The listing builds one solid part. Answer for the finished solid, in the listing's coordinates (mm). Face numbers are marked on the shaded views. A direction names the side the tool comes from. Coordinates: 2 decimals unless noted, no trailing zeros. Order: outer loops, then holes, each group sorted by start corner. A loop starts at its lowest first (then second) coordinate and runs counter-clockwise, first axis right, second up. Notation, with made-up numbers: (1.5, 4.5) -> (44.5, 4.5) arc R15 ccw to (44.5, 11.5) -> close; hole circle Ø8 at (-22.75, 55). An arc over 180 degrees is marked (long way). One line per question, with ' | ' between items.
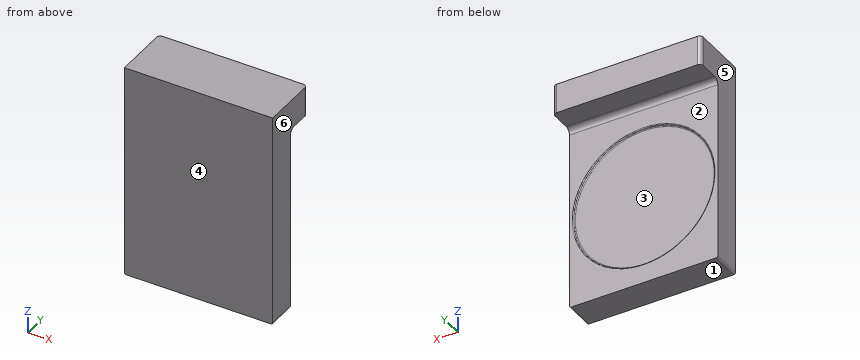
from build123d import *

# Parameters (mm, degrees)
SKETCH1_W           = 580
SKETCH1_H           = 80
BOSS_EXTRUDE1_DEPTH = 400
SKETCH2_W           = 400
SKETCH2_H           = 80
BOSS_EXTRUDE2_DEPTH = 75
FILLET2_R           = 10
FILLET3_R           = 5
FILLET4_R           = 15
SKETCH3_R           = 190
CUT_EXTRUDE1_DEPTH  = 5
FILLET6_R           = 2.5


with BuildPart() as part:
    # Sketch1 → Boss-Extrude1 (new body)
    with BuildSketch(Plane(origin=(0, 0, 0), x_dir=(0, 0, -1), z_dir=(1, 0, 0))):
        with Locations((290, 40)):
            Rectangle(SKETCH1_W, SKETCH1_H)
    extrude(amount=BOSS_EXTRUDE1_DEPTH)

    # Sketch2 → Boss-Extrude2 (add)
    with BuildSketch(Plane(origin=(0, 80, 0), x_dir=(1, 0, 0), z_dir=(0, 1, 0))):
        with Locations((200, 40)):
            Rectangle(SKETCH2_W, SKETCH2_H)
    extrude(amount=BOSS_EXTRUDE2_DEPTH)

    # Fillet2
    fillet2_edges = [part.edges().sort_by_distance(p)[0] for p in [
        (0, 155, -40),
        (400, 155, -40),
    ]]
    fillet(fillet2_edges, radius=FILLET2_R)

    # Fillet3
    fillet3_edges = [part.edges().sort_by_distance(p)[0] for p in [
        (400, 40, -580),
        (0, 40, -580),
    ]]
    fillet(fillet3_edges, radius=FILLET3_R)

    # Fillet4
    fillet4_edges = [part.edges().sort_by_distance(p)[0] for p in [
        (200, 80, -80),
    ]]
    fillet(fillet4_edges, radius=FILLET4_R)

    # Sketch3 → Cut-Extrude1 (cut)
    with BuildSketch(Plane(origin=(0, 80, 0), x_dir=(1, 0, 0), z_dir=(0, 1, 0))):
        with Locations(Location((200, 337.5, 0), (0, 0, 270))):
            Circle(SKETCH3_R)
    extrude(amount=-CUT_EXTRUDE1_DEPTH, mode=Mode.SUBTRACT)

    # Fillet6
    fillet6_edges = [part.edges().sort_by_distance(p)[0] for p in [
        (200, 75, -527.5),
        (200, 80, -527.5),
    ]]
    fillet(fillet6_edges, radius=FILLET6_R - 0.0001)  # a hair under: the kernel refuses the full size


solid = part.part
Item 1: Each of these flat-tipped pins is pushed along its axis until it touches: pin 1 Ø5 at (x, z) = (109, -120.5) entering from +Y; pin 2 Ø10 at (x, y) = (128, 94.5) entering from -Z. Where does it stop, or does it pass through?
Computed values:
pin 1: stops at y = 80 | pin 2: stops at z = -81.04
Item 2: Determine the mould class of the marked faces 3, 4, 5 and 6 for opening direction X: pulls with the +X half, pulls with the -X half, needs draft (parallel to the pull), parting line crosses it, or undercut.
Computed values:
face 3: undercut | face 4: needs draft | face 5: pulls with the -X half | face 6: pulls with the +X half
Item 3: For the marked faces 1 and 2, determine the directions among +Z, -Z, +X, -X, +Y, -Y from which every point of the face is accessible in a straight line to the end or side of a thin tool.
Computed values:
face 1: -Z, +X, -X, +Y, -Y | face 2: -Z, +X, -X, +Y
Item 4: Section C-C, the plane y = 123 is taken. Give the vertices of the cut face in (x, z).
Computed values:
outline: (0, -80) -> (400, -80) -> (400, 0) -> (0, 0) -> close
Item 5: Find the intervals of material crossed by L1, parallel to X at y = 77.55, z = -337.5; L2, parallel to X at y = 77, z = -337; L3, parallel to Y at x = 224, z = -514.5, in increasing order.
Computed values:
L1: x = 0 to 10, 390 to 400 | L2: x = 0 to 10.05, 389.95 to 400 | L3: y = 0 to 75
Item 6: Section D-D, the plane y = 88.5 is taken. Give the vertices of the cut face in (x, z).
Computed values:
outline: (0, -81.48) -> (400, -81.48) -> (400, 0) -> (0, 0) -> close
